Here's how the part is built. I have some questions about the finished solid (model axes, mm). A direction names the side the tool comes from. Give positions to 0.01 mm unless a question says otherwise; leave off trailing zeros. Write each loop counter-clockwise with the first axis right and the second up, starting at its lowest first coordinate (ties: lowest second). Pieces come first, ordered by that corner, then holes. Notation, with made-up numbers: (39.5, 70.5) -> (82.5, 70.5) arc R10 ccw to (82.5, 80.5) -> close; hole circle Ø4 at (77, 9). An arc over 180 degrees is marked (long way). Use one line per item in the form item = value.
```python
from build123d import *

# Parameters (mm, degrees)
SKETCH2_R               = 2.4
BOSS_EXTRUDE1_DEPTH     = 25
BOSS_EXTRUDE4_DEPTH     = 4.9
SKETCH5_R               = 1
CUT_EXTRUDE2_DEPTH      = 1
CUT_EXTRUDE2_DEPTH_BACK = 5.8


with BuildPart() as part:
    # Sketch2 → Boss-Extrude1 (new body, symmetric)
    with BuildSketch(Plane(origin=(0, 0, 0), x_dir=(0, 0, -1), z_dir=(1, 0, 0))):
        Circle(SKETCH2_R)
    extrude(amount=BOSS_EXTRUDE1_DEPTH, both=True)

    # Sketch3 → Boss-Extrude4 (add)
    with BuildSketch(Plane.ZY.offset(25)):
        with BuildLine():
            Line((0, 2.4), (-2.408318916, 2.4))
            ThreePointArc((-2.408318916, 2.4), (-3.4, 0), (-2.408318916, -2.4))
            Line((-2.408318916, -2.4), (0, -2.4))
            ThreePointArc((0, -2.4), (-2.4, 0), (0, 2.4))
        make_face()
        with BuildLine():
            Line((2.408318916, 2.4), (0, 2.4))
            ThreePointArc((0, 2.4), (1.697056275, 1.697056275), (2.4, 0))
            ThreePointArc((2.4, 0), (1.697056275, -1.697056275), (0, -2.4))
            Line((0, -2.4), (2.408318916, -2.4))
            ThreePointArc((2.408318916, -2.4), (3.142314777, -1.298405885), (3.4, 0))
            ThreePointArc((3.4, 0), (3.142314777, 1.298405885), (2.408318916, 2.4))
        make_face()
    extrude(amount=-BOSS_EXTRUDE4_DEPTH)

    # Sketch5 → Cut-Extrude2 (cut, two sides)
    with BuildSketch(Plane(origin=(0, 2.4, 0), x_dir=(1, 0, 0), z_dir=(0, 1, 0))) as cut_extrude2_sk:
        with Locations((22.55, -0.1)):
            Circle(SKETCH5_R)
    extrude(amount=CUT_EXTRUDE2_DEPTH, mode=Mode.SUBTRACT)
    extrude(cut_extrude2_sk.sketch, amount=-CUT_EXTRUDE2_DEPTH_BACK, mode=Mode.SUBTRACT)


solid = part.part
```
Q1. Which directions (+Z, -Z, +X, -X, +Y, -Y) give clear straight access to the entire face, cutting with the end or side of a thin tool? Please do faces 1 (the face through (-20.1, 0, -3)), 2 (the face through (-20.1, 0, 3)), 3 (the face through (-23, 2.4, 0)), 4 (the face through (25, 0, 0)), 5 (the face through (2.77, 0.72, -2.29)).
Result set:
face_1 = -Z, +X
face_2 = +Z, +X
face_3 = +Z, -Z, +X, -X, +Y
face_4 = +Z, -Z, +X, +Y, -Y
face_5 = +X
Q2. I want a section at A-A, the plane y = 0.75. Write out the boundary of the cut face in (x, z).
Result set:
outline = (-25, -3.32) -> (-20.1, -3.32) -> (-20.1, -2.28) -> (25, -2.28) -> (25, 2.28) -> (-20.1, 2.28) -> (-20.1, 3.32) -> (-25, 3.32) -> close; hole circle Ø2 at (22.55, 0.1)
Q3. If I drill on line 1 along X through (y, z) = (1.3, 0.1); line 2 along Z through (x, y) = (22.55, 0.55); line 3 along Z through (x, y) = (22.55, -1.2), over which ranges is the centre line in solid material (lowest first)? Write a range as from..to.
Result set:
line_1 = -25..21.55, 23.55..25
line_2 = -2.34..-0.9, 1.1..2.34
line_3 = -2.08..-0.9, 1.1..2.08
Q4. If we mould it in two halves opening along X, with no side actions, what happens to faces 6 (the face through (-23, -2.4, 0)), 7 (the face through (22.42, 0.03, -0.89)), 8 (the face through (-25, 0, 0))? For each: +X half, -X half, draft (parallel to the pull), parting line (faces both ways), or undercut.
Result set:
face_6 = draft
face_7 = undercut
face_8 = -X half
Q5. Will these pins go through, and if not, where does the flat tip stop? pin 1 Ø2 at (x, y) = (-10, -1) entering from +Z; pin 2 Ø1.5 at (x, y) = (-3.5, -1.5) entering from +Z; pin 3 Ø1.5 at (x, y) = (17.5, 2) entering from +Z.
Result set:
pin_1 = 2.4
pin_2 = 2.28
pin_3 = 2.05
Q6. I want a section at C-C, the plane x = -2.5. Write out the boundary of the cut face in (y, z).
Result set:
outline = circle Ø4.8 at (0, 0)
Q7. I want a section at B-B, the plane x = 22.55. Write out the boundary of the cut face in (y, z), and give its area (3 significant figures).
Result set:
outline = (-2.22, -0.9) arc R2.4 ccw to (2.22, -0.9) -> close; (-2.13, 1.1) -> (2.13, 1.1) arc R2.4 ccw to start
area = 8.79 mm2
